Can you work these out from the drawing? Everything is in mm from the part's minimum corner. A direction names the side the tool comes from. Give positions to 0.01 mm unless a question says otherwise; leave off trailing zeros. Order: outer loops, then holes, each group sorted by start corner. A loop starts at its lowest first (then second) coordinate and runs counter-clockwise, first axis right, second up. Notation, with made-up numbers: M 46,17 L 87,17 A32 cw 87,50 Z; hole C -17,-20 d10. An arc over 180 degrees is marked long. Answer in a Markdown table with one row per item. Add a question column.
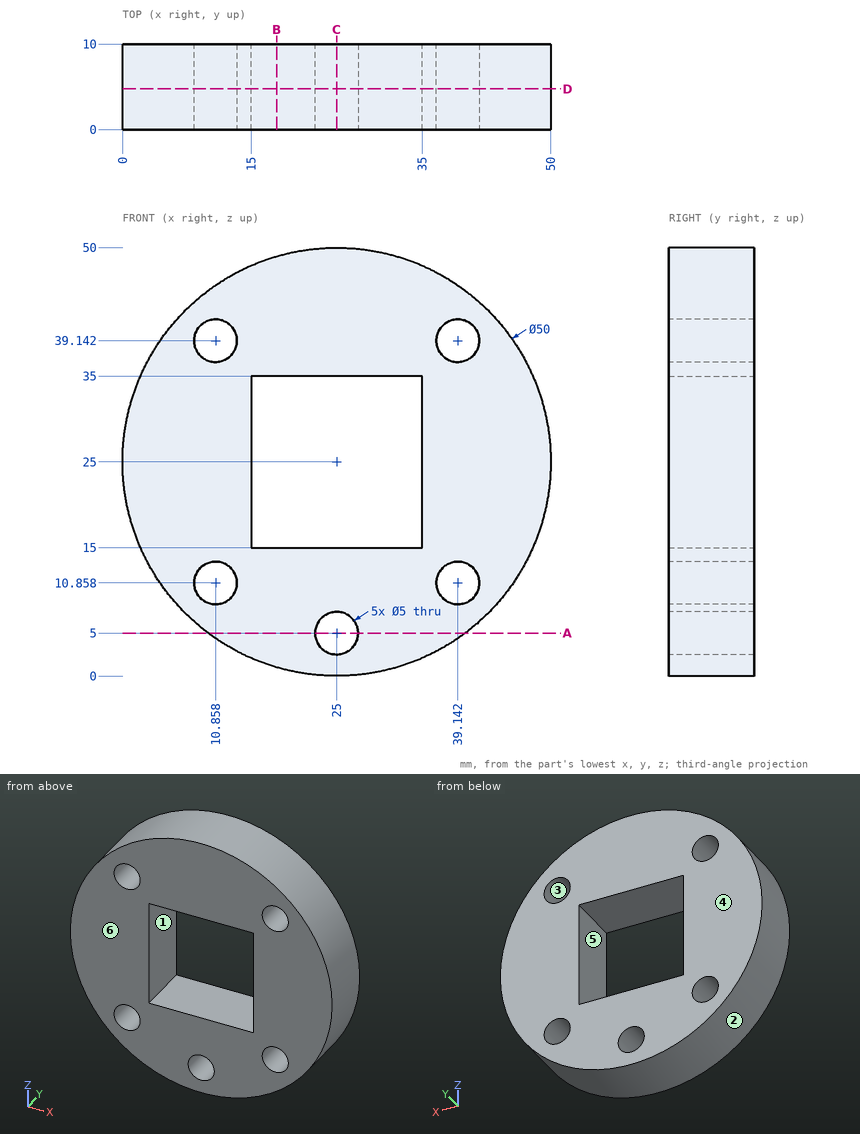
1. Suppose I cut it at A-A on z = 5. List the corners of the cut face in (x, y) for me, plus the area to 3 significant figures.
2. For the marked faces 5 and 6, which set-ups out of +Z, -Z, +X, -X, +Y, -Y let a thin tool reach every point of the face, with its end or its side?
3. Suppose I cut it at C-C on x = 25. List the corners of the cut face in (y, z) for me, plus the area to 3 significant figures.
4. If I drill on line 1 along X through (y, z) = (3.5, 41) (1 decimal); line 2 along Z through (x, y) = (23.5, 5.75) (1 decimal); line 3 along Z through (x, y) = (33, 6), over which ranges is the centre line in solid material (lowest first)? Write a range as [from, to].
5. Thinking about a two-plate mould opening in Z: for the marked faces 1, 2, 3 and 4, which applies, pulls with the +Z half, pulls with the -Z half, needs draft (parallel to the pull), parting line crosses it, or undercut?
6. Suppose I cut it at D-D on y = 4.75. List the corners of the cut face in (x, z) for me.
7. Will these pins go through, and if not, where does the flat tip stop? P1, Ø2, axis at y = 3, z = 20, coming from the +X side; P2, Ø6, axis at x = 12, y = 8.5, coming from the +Z side; P3, Ø1.5, axis at x = 35, y = 5, coming from the -Z side.
8. Suppose I cut it at B-B on x = 18. List the corners of the cut face in (y, z) for me, plus the area to 3 significant figures.
Findings below:
| question | item | result |
|---|---|---|
| 1 | outline | M 10,0 L 22.5,0 L 22.5,10 L 10,10 Z; M 27.5,0 L 40,0 L 40,10 L 27.5,10 Z |
| 1 | area | 250 mm2 |
| 2 | face 5 | +Y, -Y |
| 2 | face 6 | +Z, -Z, +X, -X, -Y |
| 3 | outline | M 0,0 L 10,0 L 10,2.5 L 0,2.5 Z; M 0,7.5 L 10,7.5 L 10,15 L 0,15 Z; M 0,35 L 10,35 L 10,50 L 0,50 Z |
| 3 | area | 250 mm2 |
| 4 | line 1 | [5.8, 9.2], [12.5, 37.5], [40.8, 44.2] |
| 4 | line 2 | [0, 3], [7, 15], [35, 50] |
| 4 | line 3 | [1.31, 15], [35, 48.69] |
| 5 | face 1 | undercut |
| 5 | face 2 | parting line crosses it |
| 5 | face 3 | undercut |
| 5 | face 4 | needs draft |
| 6 | outline | C 25,25 d50; hole C 10.86,10.86 d5; hole C 10.86,39.14 d5; hole M 15,15 L 35,15 L 35,35 L 15,35 Z; hole C 25,5 d5; hole C 39.14,10.86 d5; hole C 39.14,39.14 d5 |
| 7 | P1 | x = 49.68 |
| 7 | P2 | z = 47.91 |
| 7 | P3 | z = 1.77 |
| 8 | outline | M 0,1 L 10,1 L 10,15 L 0,15 Z; M 0,35 L 10,35 L 10,49 L 0,49 Z |
| 8 | area | 280 mm2 |
